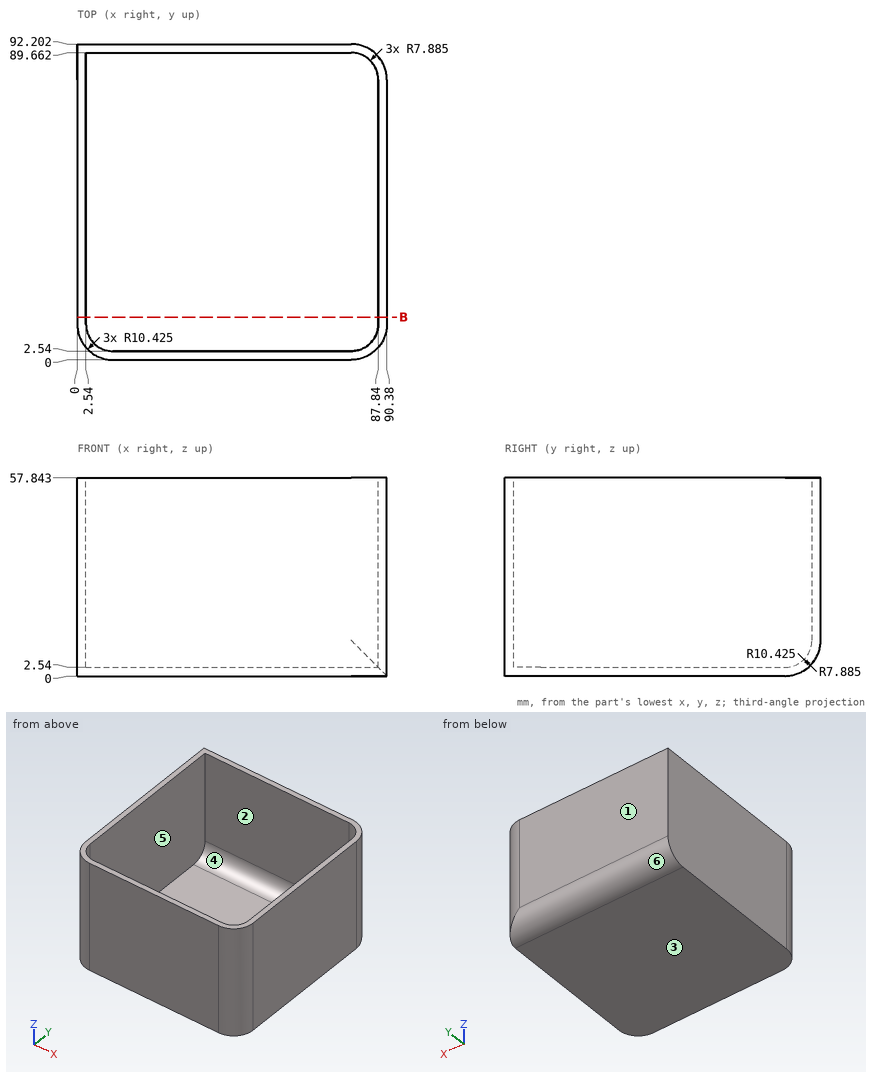
Verification items for this drawing (mm, ordinates from the low corner). A direction names the side the tool comes from. Round coordinates to 2 decimals unless told otherwise and drop trailing zeros. Loops run counter-clockwise (first coordinate to the right, second up) from the corner with the lowest first, then second, coordinate; pieces in that order, holes last. Notation, with made-up numbers: (38.5, -5) -> (49.5, -5) arc R36 cw to (49.5, 31) -> close; hole circle Ø2 at (27, 45). An arc over 180 degrees is marked (long way). Write item = value, one per line. Start each with the question number.
1) Thickness scan on probe 1 along X at (y, z) = (44.5, 52); probe 2 along Y at (x, z) = (31.5, 11); probe 3 along Z at (x, y) = (30, 66). Record the ranges inside material, lowest first.
2) Sectioned sample at B-B, the plane y = 12.5. Record the cut outline in (x, z).
3) Set-up check for the marked faces 1 and 2: record each of +Z, -Z, +X, -X, +Y, -Y from which the full face is reachable in a straight line by a thin tool's end or side.
4) Release check for a two-part mould opening along Y. For the marked faces 3, 4, 5 and 6 record: released by +Y, released by -Y, zero draft, split by the parting line, or undercut.
5) Gauge pin test, flat end, axial feed: pin 1 Ø2 at (x, y) = (64, 42) entering from +Z. Record the tip position at first contact, or that the pin passes through.
Results are:
q1.probe_1 = 0 to 2.54, 87.84 to 90.38
q1.probe_2 = 0 to 2.54, 89.66 to 92.2
q1.probe_3 = 0 to 2.54
q2.outline = (0, 0) -> (90.38, 0) -> (90.38, 57.84) -> (87.84, 57.84) -> (87.84, 2.54) -> (2.54, 2.54) -> (2.54, 57.84) -> (0, 57.84) -> close
q3.face_1 = +Z, -Z, +X, -X, +Y
q3.face_2 = +Z
q4.face_3 = zero draft
q4.face_4 = undercut
q4.face_5 = undercut
q4.face_6 = released by +Y
q5.pin_1 = 2.54
